Answer from the drawing. Dimensions are ordinates in mm from the lowest x, y and z of the part. Coordinates: 2 decimals unless noted, no trailing zeros. Order: outer loops, then holes, each group sorted by start corner. A loop starts at its lowest first (then second) coordinate and runs counter-clockwise, first axis right, second up. Notation, with made-up numbers: (0, 33) -> (23, 33) arc R14 cw to (23, 52) -> close; hole circle Ø11 at (56.5, 45). An arc over 180 degrees is marked (long way). Answer in a Markdown table with one row per item.
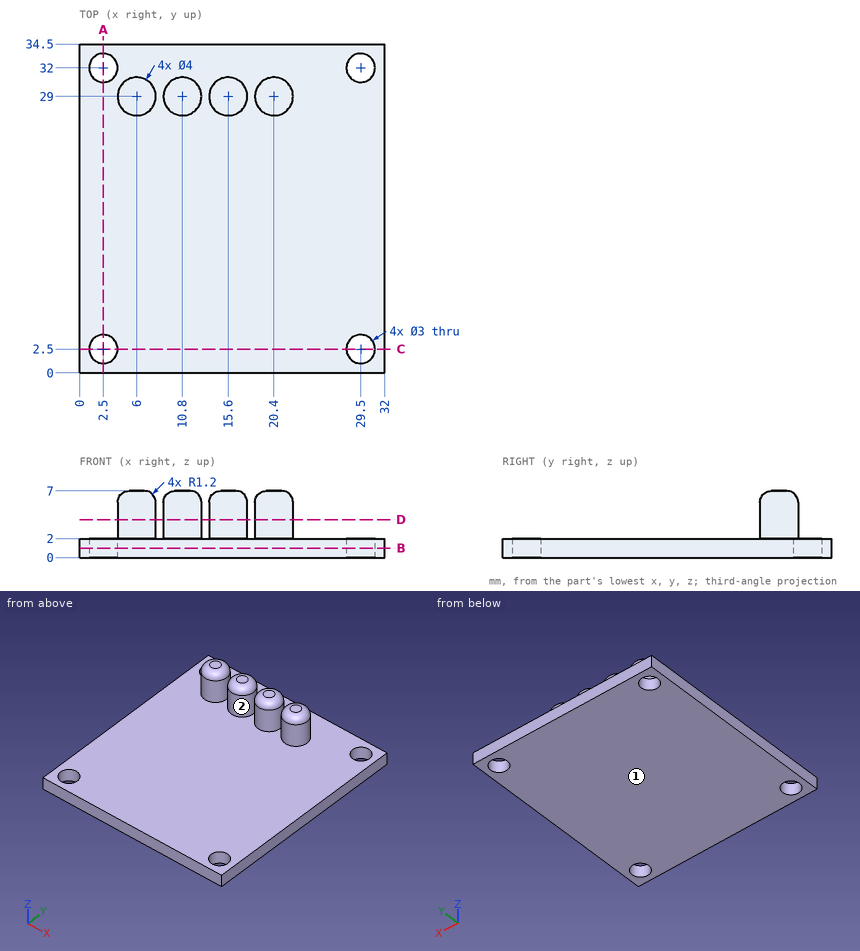
Q1. The part is cut by section B-B (z = 1). Write down the section's boundary in (x, y), then the cut area to 3 significant figures.
Outcome:
| item | result |
|---|---|
| outline | (0, 0) -> (32, 0) -> (32, 34.5) -> (0, 34.5) -> close; hole circle Ø3 at (2.5, 2.5); hole circle Ø3 at (2.5, 32); hole circle Ø3 at (29.5, 2.5); hole circle Ø3 at (29.5, 32) |
| area | 1,080 mm² |
Q2. Consider line 1 (Y direction, x = 29.5, z = 0.75); line 2 (X direction, y = 31, z = 1); line 3 (Z direction, x = 13.5, y = 12.5). Determine where each line is inside the solid, lowest interval first.
Outcome:
| item | result |
|---|---|
| line 1 | 0 to 1, 4 to 30.5, 33.5 to 34.5 |
| line 2 | 0 to 1.38, 3.62 to 28.38, 30.62 to 32 |
| line 3 | 0 to 2 |
Q3. For a pull along X with two mould halves and no side action, classify the marked faces 1 and 2 as pulls with the +X half, pulls with the -X half, needs draft (parallel to the pull), parting line crosses it, or undercut.
Outcome:
| item | result |
|---|---|
| face 1 | needs draft |
| face 2 | undercut |
Q4. The part is cut by section C-C (y = 2.5). Write down the section's boundary in (x, z), then the cut area to 3 significant figures.
Outcome:
| item | result |
|---|---|
| outline | (0, 0) -> (1, 0) -> (1, 2) -> (0, 2) -> close; (4, 0) -> (28, 0) -> (28, 2) -> (4, 2) -> close; (31, 0) -> (32, 0) -> (32, 2) -> (31, 2) -> close |
| area | 52.0 mm² |
Q5. The part is cut by section A-A (x = 2.5). Write down the section's boundary in (y, z).
Outcome:
| item | result |
|---|---|
| outline | (0, 0) -> (1, 0) -> (1, 2) -> (0, 2) -> close; (4, 0) -> (30.5, 0) -> (30.5, 2) -> (4, 2) -> close; (33.5, 0) -> (34.5, 0) -> (34.5, 2) -> (33.5, 2) -> close |
Q6. Given pin 1 (1.5 mm diameter, centred on y = 29, z = 4.5, fed in from -X); pin 2 (2.5 mm diameter, centred on x = 2.5, y = 32, fed in from -Z), each flat-ended and moving along its own axis, determine where each tip first touches the part or whether it passes through.
Outcome:
| item | result |
|---|---|
| pin 1 | x = 4 |
| pin 2 | through |
Q7. The part is cut by section D-D (z = 4). Write down the section's boundary in (x, y), then the cut area to 3 significant figures.
Outcome:
| item | result |
|---|---|
| outline | circle Ø4 at (6, 29); circle Ø4 at (10.8, 29); circle Ø4 at (15.6, 29); circle Ø4 at (20.4, 29) |
| area | 50.3 mm² |
